Can you work these out from the model? Positions are in its coordinate system, mm. Face numbers are marked on the shaded views. A direction names the side the tool comes from. Give positions to 0.01 mm unless a question says otherwise; leave off trailing zeros. Order: outer loops, then holes, each group sorted by start corner. A loop starts at its lowest first (then second) coordinate and runs counter-clockwise, first axis right, second up. Notation, with made-up numbers: (72, 49) -> (88, 49) arc R15 cw to (88, 65) -> close; hole circle Ø3 at (78.25, 21.5). An arc over 180 degrees is marked (long way). Answer as a JSON object with one key per item and string values.
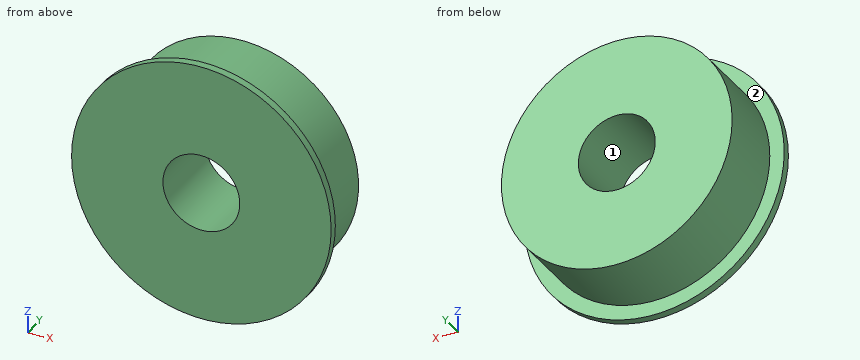
Autodesk Inventor part; units mm, degrees
ref_plane "YZ Plane" through (0, 0, 0) normal (1, 0, 0) x (0, 1, 0)
ref_plane "XZ Plane" through (0, 0, 0) normal (0, 1, 0) x (-1, 0, 0)
ref_plane "XY Plane" through (0, 0, 0) normal (0, 0, 1) x (1, 0, 0)
sketch "Sketch1" plane through (0, 0, 0) normal (0, 1, 0) x (-1, 0, 0)
  circle A0 centre (0, 0) radius 13.5
  circle A1 centre (0, 0) radius 12
  circle A2 centre (0, 0) radius 4
  dimension "d0" = 27
  dimension "d1" = 24
  dimension "d2" = 8
extrude "Extrusion1" add sketch "Sketch1" along normal blind 8 contours A1
extrude "Extrusion2" add sketch "Sketch1" along normal blind 0.8 contours A0 | A1 | A2
extrude "Extrusion3" cut sketch "Sketch1" along normal blind 0.8 contours A2
properties part number "FlangedBearing"
1. If we section it at D-D on z = 6.5: Please give me the cut outline in (x, y).
Worked answers:
{"outline": "(-11.83, 0) -> (11.83, 0) -> (11.83, 0.8) -> (10.09, 0.8) -> (10.09, 8) -> (-10.09, 8) -> (-10.09, 0.8) -> (-11.83, 0.8) -> close"}
2. Will these pins go through, and if not, where does the flat tip stop? pin 1 Ø10 at (x, z) = (2.5, 6.5) entering from -Y; pin 2 Ø4 at (y, z) = (2.5, -5.5) entering from -X.
Worked answers:
{"pin 1": "y = 0", "pin 2": "x = -12.75"}
3. If we section it at B-B on x = 0: Please give me the cut outline in (y, z).
Worked answers:
{"outline": "(0, -13.5) -> (0.8, -13.5) -> (0.8, -12) -> (8, -12) -> (8, -4) -> (0, -4) -> close; (0, 4) -> (8, 4) -> (8, 12) -> (0.8, 12) -> (0.8, 13.5) -> (0, 13.5) -> close"}
4. Please list where these lines run through material, in increasing order: L1, parallel to Z at x = -0.25, y = 0.5; L2, parallel to Y at x = -6.75, z = -11; L3, parallel to Z at x = 0, y = 3.5.
Worked answers:
{"L1": "-13.5 to -3.99, 3.99 to 13.5", "L2": "0 to 0.8", "L3": "-12 to -4, 4 to 12"}
5. For the marked faces 1 and 2, which set-ups out of +Z, -Z, +X, -X, +Y, -Y let a thin tool reach every point of the face, with its end or its side?
Worked answers:
{"face 1": "+Y, -Y", "face 2": "+Y"}
6. If we section it at C-C on y = 2.75: Please give me the cut outline in (x, z), then the cut area to 3 significant figures.
Worked answers:
{"outline": "circle Ø24 at (0, 0); hole circle Ø8 at (0, 0)", "area": "402 mm²"}
7. If we section it at A-A on z = 0: Please give me the cut outline in (x, y).
Worked answers:
{"outline": "(-13.5, 0) -> (-4, 0) -> (-4, 8) -> (-12, 8) -> (-12, 0.8) -> (-13.5, 0.8) -> close; (4, 0) -> (13.5, 0) -> (13.5, 0.8) -> (12, 0.8) -> (12, 8) -> (4, 8) -> close"}
